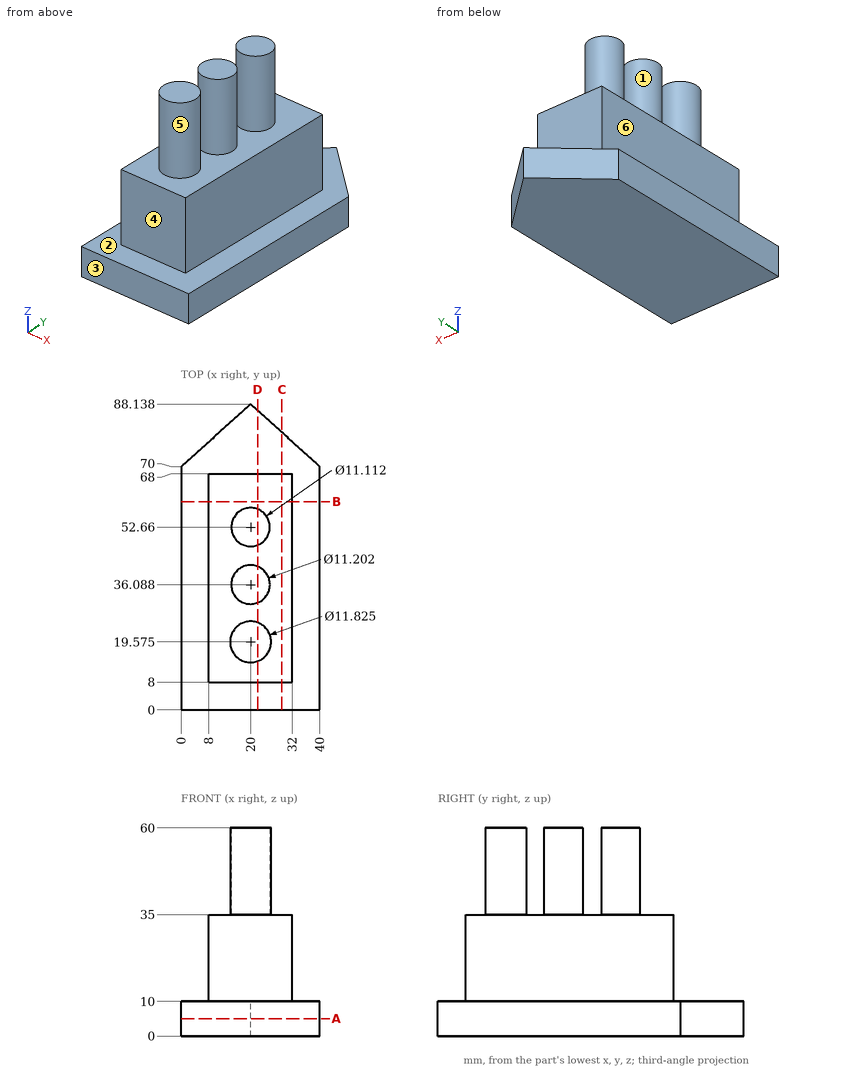
Study the drawing (mm; zero at the part's minimum x, y, z) and answer. A direction names the side the tool comes from. Give positions to 0.01 mm unless a question says otherwise; leave off trailing zeros. Order: outer loops, then holes, each group sorted by start corner. A loop starts at its lowest first (then second) coordinate and runs counter-clockwise, first axis right, second up. Notation, with made-up numbers: (-23.75, 7.5) - (19.25, 7.5) arc R27 ccw to (19.25, 45.5) - close; hole circle Ø6 at (-9.5, -29.75). An arc over 180 degrees is marked (long way). Use one line per item in the form item = value. Start each with the question number.
(1) Flat-ended cylindrical pins translate along their axes: pin 1 Ø8 at (x, z) = (22.5, 30) entering from +Y; pin 2 Ø6 at (y, z) = (63.5, 35) entering from -X; pin 3 Ø7.5 at (y, z) = (49, 26.5) entering from +X; pin 4 Ø10 at (x, y) = (26, 42.5) entering from -Z. Find the tip coordinate at first contact, or state that the pin passes through.
(2) A cutting plane is placed at A-A, the plane z = 5. Write down the section's boundary in (x, y).
(3) A cutting plane is placed at D-D, the plane x = 22. Write down the section's boundary in (y, z) (1 decimal).
(4) Consider line 1 (Y direction, x = 23.5, z = 48) (1 decimal); line 2 (Y direction, x = 16, z = 49.5) (1 decimal); line 3 (X direction, y = 47.5, z = 33.5). Determine where each line is inside the solid, lowest interval first. Write a range as from..to.
(5) For the marked faces 4, 5 and 6, determine the directions among +Z, -Z, +X, -X, +Y, -Y from which every point of the face is accessible in a straight line to the end or side of a thin tool.
(6) A cutting plane is placed at B-B, the plane y = 60. Write down the section's boundary in (x, z), then the cut area to 3 significant figures.
(7) The mould has two halves that part along Y. Classify the marked faces 1, 2 and 3: released by +Y, released by -Y, zero draft, split by the parting line, or undercut.
(8) A cutting plane is placed at C-C, the plane x = 29. Write down the section's boundary in (y, z).
Ans:
q1.pin_1 = 68
q1.pin_2 = 8
q1.pin_3 = 32
q1.pin_4 = 0
q2.outline = (0, 0) - (40, 0) - (40, 70) - (20, 88.14) - (0, 70) - close
q3.outline = (0, 0) - (86.3, 0) - (86.3, 10) - (68, 10) - (68, 35) - (57.8, 35) - (57.8, 60) - (47.5, 60) - (47.5, 35) - (41.3, 35) - (41.3, 60) - (30.9, 60) - (30.9, 35) - (25.1, 35) - (25.1, 60) - (14, 60) - (14, 35) - (8, 35) - (8, 10) - (0, 10) - close
q4.line_1 = 14.8..24.3, 31.7..40.5, 48.3..57
q4.line_2 = 15.2..23.9, 32.2..40, 48.8..56.5
q4.line_3 = 8..32
q5.face_4 = +Z, +X, -X, -Y
q5.face_5 = +Z
q5.face_6 = +Z, -X, +Y, -Y
q6.outline = (0, 0) - (40, 0) - (40, 10) - (32, 10) - (32, 35) - (8, 35) - (8, 10) - (0, 10) - close
q6.area = 1,000 mm^2
q7.face_1 = undercut
q7.face_2 = zero draft
q7.face_3 = released by -Y
q8.outline = (0, 0) - (79.98, 0) - (79.98, 10) - (68, 10) - (68, 35) - (8, 35) - (8, 10) - (0, 10) - close
